```python
from build123d import *

# Parameters (mm, degrees)
F0_R     = 50.8
F0_R_2   = 25.4
F0_R_3   = 12.7
F2_DEPTH = 76.2
F3_DEPTH = 152.4
F4_DEPTH = 281.178
F5_SIZE  = 8.89
F1_W     = 406.4
F1_H     = 25.4
F6_DEPTH = 715.518


with BuildPart() as f2:
    # F0 (on Top) → F2 (new body)
    with BuildSketch(Plane.XY):
        with BuildLine():
            Line((101.6, 0), (-101.6, 0))
            ThreePointArc((-101.6, 0), (-304.8, -203.2), (-101.6, -406.4))
            Line((-101.6, -406.4), (101.6, -406.4))
            ThreePointArc((101.6, -406.4), (304.8, -203.2), (101.6, 0))
        make_face()
        with BuildLine():
            ThreePointArc((-101.6, -330.2), (-228.6, -203.2), (-101.6, -76.2))
            Line((-101.6, -76.2), (101.6, -76.2))
            ThreePointArc((101.6, -76.2), (228.6, -203.2), (101.6, -330.2))
            Line((101.6, -330.2), (-101.6, -330.2))
        make_face(mode=Mode.SUBTRACT)
        with BuildLine():
            Line((101.6, -76.2), (-101.6, -76.2))
            ThreePointArc((-101.6, -76.2), (-228.6, -203.2), (-101.6, -330.2))
            Line((-101.6, -330.2), (101.6, -330.2))
            ThreePointArc((101.6, -330.2), (228.6, -203.2), (101.6, -76.2))
        make_face()
        with BuildLine():
            ThreePointArc((101.6, -133.35), (171.45, -203.2), (101.6, -273.05))
            Line((101.6, -273.05), (-101.6, -273.05))
            ThreePointArc((-101.6, -273.05), (-171.45, -203.2), (-101.6, -133.35))
            Line((-101.6, -133.35), (101.6, -133.35))
        make_face(mode=Mode.SUBTRACT)
        with BuildLine():
            Line((-101.6, -273.05), (101.6, -273.05))
            ThreePointArc((101.6, -273.05), (171.45, -203.2), (101.6, -133.35))
            Line((101.6, -133.35), (-101.6, -133.35))
            ThreePointArc((-101.6, -133.35), (-171.45, -203.2), (-101.6, -273.05))
        make_face()
        with Locations((-101.6, -203.2)):
            Circle(F0_R, mode=Mode.SUBTRACT)
        with Locations((101.6, -203.2)):
            Circle(F0_R, mode=Mode.SUBTRACT)
        with Locations((101.6, -203.2)):
            Circle(F0_R)
        with Locations((101.6, -203.2)):
            Circle(F0_R_2, mode=Mode.SUBTRACT)
        with Locations((-101.6, -203.2)):
            Circle(F0_R)
        with Locations((-101.6, -203.2)):
            Circle(F0_R_2, mode=Mode.SUBTRACT)
        with Locations((101.6, -203.2)):
            Circle(F0_R_2)
        with Locations((101.6, -203.2)):
            Circle(F0_R_3, mode=Mode.SUBTRACT)
        with Locations((-101.6, -203.2)):
            Circle(F0_R_2)
        with Locations((-101.6, -203.2)):
            Circle(F0_R_3, mode=Mode.SUBTRACT)
        with Locations((101.6, -203.2)):
            Circle(F0_R_3)
        with Locations((-101.6, -203.2)):
            Circle(F0_R_3)
    extrude(amount=F2_DEPTH)

    # F0 (on Top) → F3 (join)
    with BuildSketch(Plane.XY):
        with BuildLine():
            Line((101.6, -76.2), (-101.6, -76.2))
            ThreePointArc((-101.6, -76.2), (-228.6, -203.2), (-101.6, -330.2))
            Line((-101.6, -330.2), (101.6, -330.2))
            ThreePointArc((101.6, -330.2), (228.6, -203.2), (101.6, -76.2))
        make_face()
        with BuildLine():
            ThreePointArc((101.6, -133.35), (171.45, -203.2), (101.6, -273.05))
            Line((101.6, -273.05), (-101.6, -273.05))
            ThreePointArc((-101.6, -273.05), (-171.45, -203.2), (-101.6, -133.35))
            Line((-101.6, -133.35), (101.6, -133.35))
        make_face(mode=Mode.SUBTRACT)
        with Locations((101.6, -203.2)):
            Circle(F0_R)
        with Locations((101.6, -203.2)):
            Circle(F0_R_2, mode=Mode.SUBTRACT)
        with Locations((-101.6, -203.2)):
            Circle(F0_R)
        with Locations((-101.6, -203.2)):
            Circle(F0_R_2, mode=Mode.SUBTRACT)
        with Locations((101.6, -203.2)):
            Circle(F0_R_2)
        with Locations((101.6, -203.2)):
            Circle(F0_R_3, mode=Mode.SUBTRACT)
        with Locations((-101.6, -203.2)):
            Circle(F0_R_2)
        with Locations((-101.6, -203.2)):
            Circle(F0_R_3, mode=Mode.SUBTRACT)
        with Locations((101.6, -203.2)):
            Circle(F0_R_3)
        with Locations((-101.6, -203.2)):
            Circle(F0_R_3)
    extrude(amount=F3_DEPTH)

    # F0 (on Top) → F4 (cut)
    with BuildSketch(Plane.XY):
        with Locations((101.6, -203.2)):
            Circle(F0_R_3)
        with Locations((-101.6, -203.2)):
            Circle(F0_R_3)
    extrude(amount=F4_DEPTH, mode=Mode.SUBTRACT)

    # F5
    f5_edges = [f2.edges().sort_by_distance(p)[0] for p in [
        (88.9, -203.2, 0),
        (114.3, -203.2, 76.2),
        (88.9, -203.2, 152.4),
        (-114.3, -203.2, 0),
        (-88.9, -203.2, 76.2),
        (-114.3, -203.2, 152.4),
    ]]
    chamfer(f5_edges, length=F5_SIZE)

    # F1 (on Front) → F6 (cut)
    with BuildSketch(Plane.XZ):
        with Locations((0, 12.7)):
            Rectangle(F1_W, F1_H)
    extrude(amount=F6_DEPTH, mode=Mode.SUBTRACT)


solid = f2.part
```
Build history of the part. All positions in model axes, mm. A direction names the side the tool comes from. Coordinates: 2 decimals unless noted, no trailing zeros. Write each loop counter-clockwise with the first axis right and the second up, starting at its lowest first coordinate (ties: lowest second). Pieces come first, ordered by that corner, then holes.
1. Drill centre lines: probe 1 along Y at (x, z) = (-101.6, 108.5); probe 2 along X at (y, z) = (-203.2, 100). Where is each one in solid material? Low to high.
Answer block:
probe 1: y = -330.2 to -273.05, -254 to -215.9, -190.5 to -152.4, -133.35 to -76.2
probe 2: x = -228.6 to -171.45, -152.4 to -114.3, -88.9 to -50.8, 50.8 to 88.9, 114.3 to 152.4, 171.45 to 228.6
2. Band-saw the part on B-B, the plane x = 29. Give the cut face in (y, z).
Answer block:
outline: (-406.4, 25.4) - (0, 25.4) - (0, 76.2) - (-76.2, 76.2) - (-76.2, 152.4) - (-133.35, 152.4) - (-133.35, 76.2) - (-273.05, 76.2) - (-273.05, 152.4) - (-330.2, 152.4) - (-330.2, 76.2) - (-406.4, 76.2) - close
3. Band-saw the part on D-D, the plane z = 67. Give the cut face in (x, y).
Answer block:
outline: (-101.6, -406.4) - (101.6, -406.4) arc R203.2 ccw to (101.6, 0) - (-101.6, 0) arc R203.2 ccw to start; hole circle Ø25.4 at (-101.6, -203.2); hole circle Ø25.4 at (101.6, -203.2)
4. 3-axis set-ups, long thin cutter, end or side, ignore diameter. For faces 1 (the cylindrical face through (228.57, -205.99, 113.77)), 2 (the flat face through (1, -76.2, 114)), 3 (the flat face through (-2, -202, 76.2)), 4 (the flat face through (203.2, -201, 13)): which of +Z, -Z, +X, -X, +Y, -Y reach the whole face in a straight line?
Answer block:
face 1: +Z, +X
face 2: +Z, +X, -X, +Y
face 3: +Z
face 4: -Z, +Y, -Y
5. Band-saw the part on C-C, the plane y = -203.2. Give the number of separate pieces and of enclosed holes in the cut face, and give its area (3 significant figures).
Answer block:
separate pieces: 3
enclosed holes: 0
area: 53,700 mm2
6. Drop flat-ended pins along their axis: pin 1 (8 mm diameter, centred on y = -159, z = 110, fed in from +X); pin 2 (8 mm diameter, centred on x = 219, y = -346, fed in from -Z); pin 3 (8 mm diameter, centred on y = -124.5, z = 83, fed in from -X); pin 4 (20.5 mm diameter, centred on y = -230.5, z = 12, fed in from +X). Give the stop position or say it passes through.
Answer block:
pin 1: stops at x = 222.07
pin 2: stops at z = 0
pin 3: stops at x = -204.31
pin 4: stops at x = 304.08
7. Pull direction X, two halves, no side cores. Call faces 5 (the cylindrical face through (-304.75, -198.73, 37.57)), 6 (the flat face through (1, 0, 50)), 7 (the cylindrical face through (-171.433, -204.736, 113.767)): released by +X, released by -X, zero draft, split by the parting line, or undercut.
Answer block:
face 5: released by -X
face 6: zero draft
face 7: undercut
8. Band-saw the part on A-A, the plane z = 109. Give the cut face in (x, y).
Answer block:
outline: circle Ø101.6 at (-101.6, -203.2); (-101.6, -330.2) - (101.6, -330.2) arc R127 ccw to (101.6, -76.2) - (-101.6, -76.2) arc R127 ccw to start; circle Ø101.6 at (101.6, -203.2); hole circle Ø25.4 at (-101.6, -203.2); hole (-101.6, -273.05) - (101.6, -273.05) arc R69.85 ccw to (101.6, -133.35) - (-101.6, -133.35) arc R69.85 ccw to start; hole circle Ø25.4 at (101.6, -203.2)
